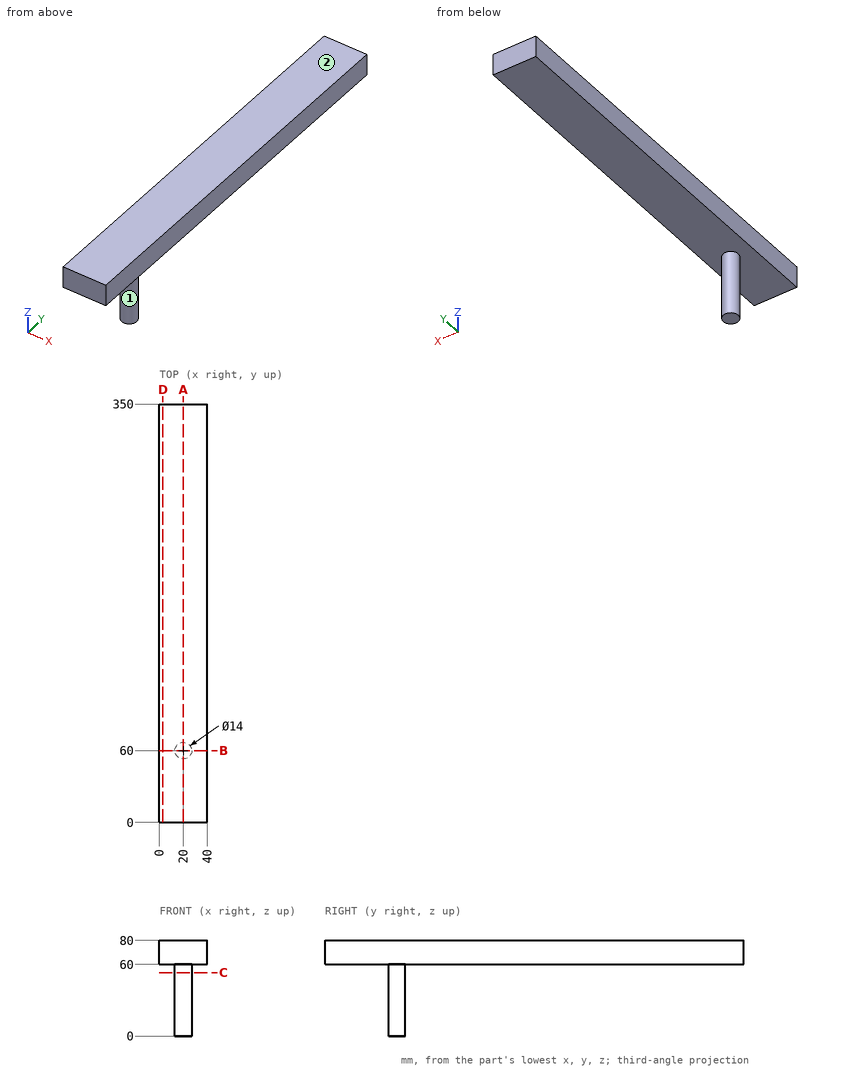
Part print with two shaded views. Sizes in mm from the minimum x, y, z corner. A direction names the side the tool comes from. Round coordinates to 2 decimals unless told otherwise and drop trailing zeros. Loops run counter-clockwise (first coordinate to the right, second up) from the corner with the lowest first, then second, coordinate; pieces in that order, holes last.
Item 1: Saw through at B-B (y = 60). List the corners of the cut face in (x, z), then the cut area to 3 significant figures.
Item 2: Pin check, flat tips, straight feed: P1, Ø8, axis at x = 6, z = 55, coming from the -Y side; P2, Ø10, axis at x = 16.5, y = 139.5, coming from the -Z side; P3, Ø5, axis at x = 25, z = 25.5, coming from the -Y side; P4, Ø5, axis at x = 28.5, z = 28.5, coming from the -Y side. Stop position of each tip, or through.
Item 3: Drill centre lines: line 1 along Z through (x, y) = (25, 51); line 2 along X through (y, z) = (59, 57); line 3 along Y through (x, z) = (25.5, 14.5). Where is each one in solid material? Low to high.
Item 4: Saw through at A-A (x = 20). List the corners of the cut face in (y, z), then the cut area to 3 significant figures.
Item 5: Saw through at D-D (x = 3). List the corners of the cut face in (y, z).
Item 6: Saw through at C-C (z = 53). List the corners of the cut face in (x, y).
Item 7: Which spindle directions (+Z, -Z, +X, -X, +Y, -Y) get a long thin tool onto all of the face, cutting with end or side? Do the marked faces 1 and 2. Say none if no direction does.
Worked answers:
1. outline: (0, 60) - (13, 60) - (13, 0) - (27, 0) - (27, 60) - (40, 60) - (40, 80) - (0, 80) - close
1. area: 1,640 mm2
2. P1: passes through
2. P2: stops at z = 60
2. P3: stops at y = 53.46
2. P4: stops at y = 56.39
3. line 1: z = 60 to 80
3. line 2: x = 13.07 to 26.93
3. line 3: y = 55.67 to 64.33
4. outline: (0, 60) - (53, 60) - (53, 0) - (67, 0) - (67, 60) - (350, 60) - (350, 80) - (0, 80) - close
4. area: 7,840 mm2
5. outline: (0, 60) - (350, 60) - (350, 80) - (0, 80) - close
6. outline: circle Ø14 at (20, 60)
7. face 1: -Z
7. face 2: +Z, +X, -X, +Y, -Y
